Autodesk Inventor part; units mm, degrees
ref_plane "YZ Plane" through (0, 0, 0) normal (1, 0, 0) x (0, 1, 0)
ref_plane "XZ Plane" through (0, 0, 0) normal (0, 1, 0) x (-1, 0, 0)
ref_plane "XY Plane" through (0, 0, 0) normal (0, 0, 1) x (1, 0, 0)
sketch "Skizze1" plane through (0, 0, 0) normal (0, 0, 1) x (1, 0, 0)
  arc A0 (0, 7) -> (0, -7) centre (0, 0) ccw
  line L0 (0, 7) -> (20, 7)
  line L1 (20, 7) -> (73.598, -46.598)
  line L2 (73.598, -46.598) -> (56.6274, -63.5685)
  line L3 (56.6274, -63.5685) -> (0.0589, -7)
  line L4 (0.0589, -7) -> (0, -7)
  line L5 (65.1127, -55.0833) -> (43.8995, -33.8701) construction
  circle A1 centre (43.8995, -33.8701) radius 6.5
  circle A2 centre (0, 0) radius 3.05
  dimension "d0" = 14
  dimension "d1" = 6.1
  dimension "d2" = 13
  dimension "d3" = 24
  dimension "d4" = 80
  dimension "d5" = 30
  dimension "d6" = 20
  dimension "d7" = 135
extrude "Extrusion1" add sketch "Skizze1" along normal blind 4
sketch "Skizze4" plane through (0, 0, 4) normal (0, 0, 1) x (1, 0, 0)
  circle A0 centre (0, 0) radius 3.05
  circle A1 centre (0, 0) radius 7
  dimension "d18" = 14
  dimension "d19" = 6.1
extrude "Extrusion4" add sketch "Skizze4" along normal blind 6
hole "Bohrung1" at (50.2635, -40.234, 4) direction (0, 0, -1) diameter 3 depth 8 tip angle 118
pattern_circular "Runde Anordnung1" count 3 over 360 about axis through (43.8995, -33.8701, 0) along (0, 0, 1) of "Bohrung1"
properties part number "Armlinks"
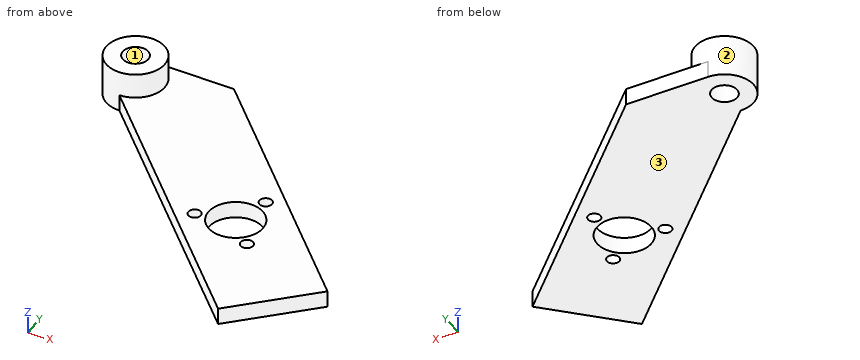
Check sheet for the modelled part. Datum: model origin and axes. Units: mm. Face numbers are marked on the shaded views. Round coordinates to 2 decimals unless told otherwise and drop trailing zeros. Order: outer loops, then holes, each group sorted by start corner. A loop starts at its lowest first (then second) coordinate and runs counter-clockwise, first axis right, second up.
(1) Cross-section at A-A, the plane y = 0. Enter the section's corners in (x, z).
(2) Draft check along X on the marked faces 1, 2 and 3. Enter one of: pulls with the +X half, pulls with the -X half, needs draft (parallel to the pull), parting line crosses it, or undercut.
(3) Cross-section at D-D, the plane x = 65. Enter the section's corners in (y, z).
(4) Scan lines: probe 1 along Y at (x, z) = (0, 4); probe 2 along Z at (x, y) = (64, -41); probe 3 along X at (y, z) = (-34.5, 0.75). Record each from-to range of solid material in increasing order.
(5) Cross-section at C-C, the plane z = 7.25. Enter the section's corners in (x, y).
(6) Go/stop test with flat-tipped pins: P1, Ø3, axis at y = -31.5, z = 5, coming from the +X side; P2, Ø1.5, axis at y = -47.5, z = 2.5, coming from the +X side; P3, Ø1.8, axis at x = 50.26, y = -40.23, coming from the +Z side; P4, Ø8, axis at x = 0, y = 0, coming from the +Z side. Record where each tip stops, or that it passes through.
(7) Cross-section at B-B, the plane z = 2.5. Enter the section's corners in (x, y), and give its area (3 significant figures).
Check sheet entries:
1. outline: (-7, 0) - (-3.05, 0) - (-3.05, 10) - (-7, 10) - close; (3.05, 0) - (27, 0) - (27, 4) - (7, 4) - (7, 10) - (3.05, 10) - close
2. face 1: undercut
2. face 2: parting line crosses it
2. face 3: needs draft
3. outline: (-55.2, 0) - (-38, 0) - (-38, 4) - (-55.2, 4) - close
4. probe 1: y = -7 to -3.05, 3.05 to 7
4. probe 2: z = 0 to 4
4. probe 3: x = 27.56 to 37.43, 50.37 to 61.5
5. outline: circle Ø14 at (0, 0); hole circle Ø6.1 at (0, 0)
6. P1: stops at x = 59.62
6. P2: stops at x = 73.45
6. P3: passes through
6. P4: stops at z = 10
7. outline: (0, -7) - (0.06, -7) - (56.63, -63.57) - (73.6, -46.6) - (20, 7) - (0, 7) arc R7 ccw to start; hole circle Ø6.1 at (0, 0); hole circle Ø3 at (35.21, -36.2); hole circle Ø13 at (43.9, -33.87); hole circle Ø3 at (46.23, -25.18); hole circle Ø3 at (50.26, -40.23)
7. area: 1,900 mm2
